Autodesk Inventor part; units mm, degrees
ref_plane "YZ Plane" through (0, 0, 0) normal (1, 0, 0) x (0, 1, 0)
ref_plane "XZ Plane" through (0, 0, 0) normal (0, 1, 0) x (-1, 0, 0)
ref_plane "XY Plane" through (0, 0, 0) normal (0, 0, 1) x (1, 0, 0)
sketch "スケッチ1" plane through (0, 0, 0) normal (0, 0, 1) x (1, 0, 0)
  circle A0 centre (0, 0) radius 2
  dimension "d0" = 4
extrude "押し出し1" add sketch "スケッチ1" along normal blind 6
sketch "スケッチ2" plane through (0, 0, 6) normal (0, 0, 1) x (1, 0, 0)
  circle A0 centre (0, 0) radius 2
  circle A1 centre (0, 0) radius 4
  dimension "d3" = 8
extrude "押し出し2" add sketch "スケッチ2" along normal blind 3 contours A0 | A1
fillet "フィレット1" radius 3 1 edges at (-4, 0, 9)
thread "ねじ1"
sketch "スケッチ3" plane through (0, 0, 0) normal (0, 0, -1) x (-1, 0, 0)
  circle A0 centre (0, 0) radius 2
extrude "押し出し3" add sketch "スケッチ3" along normal blind 19
properties part number "SB　M4 25mm なべネジ" material "Stainless Steel, 440C"
Can you work these out from the model? Positions are in its coordinate system, mm. A direction names the side the tool comes from. Round coordinates to 2 decimals unless told otherwise and drop trailing zeros. Write each loop counter-clockwise with the first axis right and the second up, starting at its lowest first coordinate (ties: lowest second). Pieces come first, ordered by that corner, then holes. Notation, with made-up numbers: (35, -2.75) - (39, -2.75) arc R19 cw to (39, 14.25) - close; hole circle Ø8 at (-16, 34). An arc over 180 degrees is marked (long way). Write each question's results on one line, items separated by ' | '. Start each with the question number.
1) For pin 1 Ø1 at (x, y) = (1, -3) entering from +Z; pin 2 Ø2 at (x, y) = (3, -0.5) entering from +Z; pin 3 Ø3 at (y, z) = (0, 3) entering from +X, each with a flat end and sliding along its axis, tell me the tip position at first contact or that it passes through.
2) Suppose I cut it at A-A (z = -10.5). List the corners of the cut face in (x, y) for me.
3) Please list where these lines run through material, in increasing order: line 1 (Z direction, x = -0.5, y = 1); line 2 (X direction, y = 0, z = 5.5); line 3 (Y direction, x = -0.25, z = 5).
4) Which directions (+Z, -Z, +X, -X, +Y, -Y) give clear straight access to the entire face, cutting with the end or side of a thin tool? Please do faces 1 (the flat face through (0, 0, 9)), 2 (the flat face through (-2, -1, 6)).
Here are the results:
1) pin 1: stops at z = 8.5 | pin 2: stops at z = 8.81 | pin 3: stops at x = 2
2) outline: circle Ø4 at (0, 0)
3) line 1: z = -19 to 9 | line 2: x = -2 to 2 | line 3: y = -1.98 to 1.98
4) face 1: +Z, +X, -X, +Y, -Y | face 2: -Z
